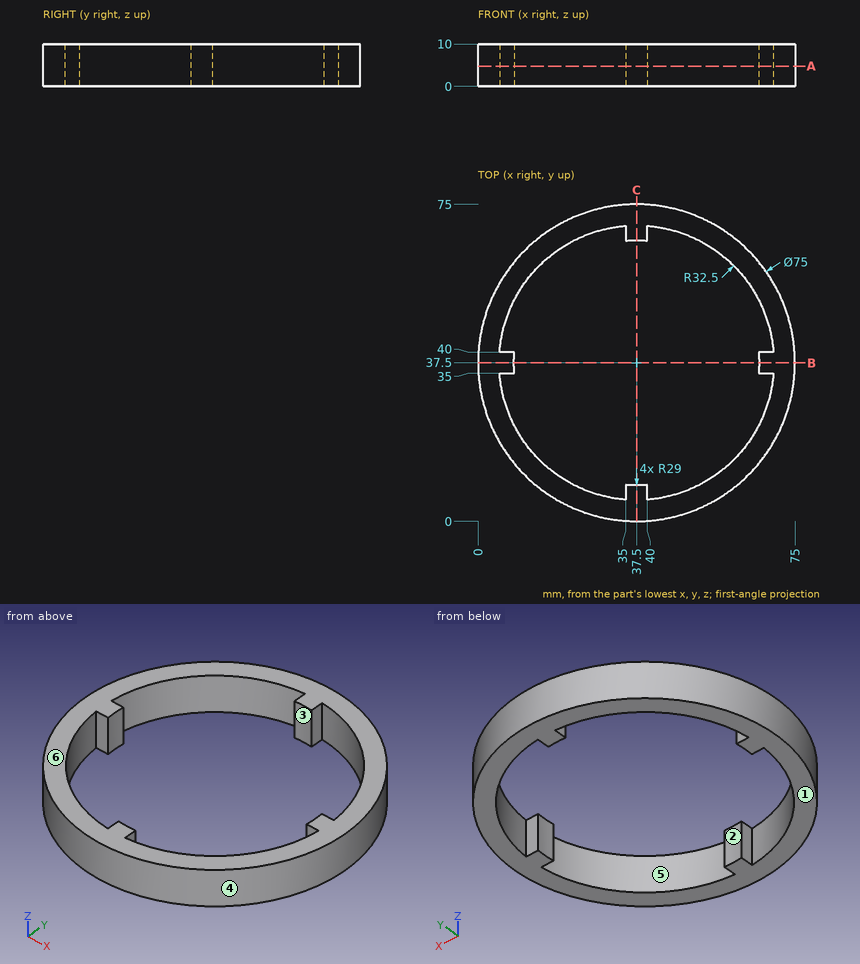
Answer from the drawing. Dimensions are ordinates in mm from the lowest x, y and z of the part. A direction names the side the tool comes from. Round coordinates to 2 decimals unless told otherwise and drop trailing zeros. Write each loop counter-clockwise with the first axis right and the second up, starting at its lowest first coordinate (ties: lowest second). Pieces come first, ordered by that corner, then holes. Notation, with made-up numbers: (13, 46.25) -> (43, 46.25) arc R34 cw to (43, 81.25) -> close; hole circle Ø8 at (-3, -23). An arc over 180 degrees is marked (long way). Answer in a Markdown table with one row per item. Add a question column.
1) Find section B-B, the plane y = 37.5. Determine the outline of the cut face in (x, z), and give its area (3 significant figures).
2) Which of the six approach directions +Z, -Z, +X, -X, +Y, -Y give full straight-line access (tool end or side, diameter ignored) to the marked faces 1 and 2?
3) Determine the mould class of the marked faces 3, 4, 5 and 6 for opening direction Y: pulls with the +Y half, pulls with the -Y half, needs draft (parallel to the pull), parting line crosses it, or undercut.
4) Given P1, Ø2, axis at x = 35.5, z = 8, coming from the +Y side; P2, Ø3, axis at x = 67.5, z = 2.5, coming from the +Y side; P3, Ø1, axis at y = 28.5, z = 7, coming from the -X side; P4, Ø3, axis at x = 13.5, y = 17, coming from the +Z side, each flat-ended and moving along its own axis, determine where each tip first touches the part or whether it passes through.
5) Consider line 1 (Y direction, x = 37, z = 2.75); line 2 (X direction, y = 32, z = 2). Determine where each line is inside the solid, lowest interval first.
6) Find section A-A, the plane z = 4.75. Determine the outline of the cut face in (x, y), and give its area (3 significant figures).
Findings below:
| question | item | result |
|---|---|---|
| 1 | outline | (0, 0) -> (8.5, 0) -> (8.5, 10) -> (0, 10) -> close; (66.5, 0) -> (75, 0) -> (75, 10) -> (66.5, 10) -> close |
| 1 | area | 170 mm² |
| 2 | face 1 | -Z, +X, -X, +Y, -Y |
| 2 | face 2 | +Z, -Z |
| 3 | face 3 | undercut |
| 3 | face 4 | parting line crosses it |
| 3 | face 5 | undercut |
| 3 | face 6 | needs draft |
| 4 | P1 | y = 74.99 |
| 4 | P2 | y = 61.87 |
| 4 | P3 | x = 0.98 |
| 4 | P4 | z = 10 |
| 5 | line 1 | 0 to 8.5, 66.5 to 75 |
| 5 | line 2 | 0.41 to 5.47, 69.53 to 74.59 |
| 6 | outline | circle Ø75 at (37.5, 37.5); hole (5.1, 35) arc R32.5 ccw to (35, 5.1) -> (35, 8.61) arc R29 ccw to (40, 8.61) -> (40, 5.1) arc R32.5 ccw to (69.9, 35) -> (66.39, 35) arc R29 ccw to (66.39, 40) -> (69.9, 40) arc R32.5 ccw to (40, 69.9) -> (40, 66.39) arc R29 ccw to (35, 66.39) -> (35, 69.9) arc R32.5 ccw to (5.1, 40) -> (8.61, 40) arc R29 ccw to (8.61, 35) -> close |
| 6 | area | 1,170 mm² |
